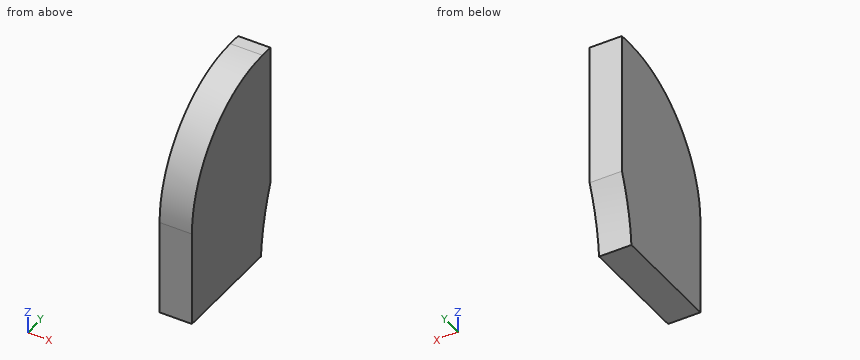
from build123d import *

# Parameters (mm, degrees)
SKETCH1_W               = 5
SKETCH1_H               = 20
BOSS_EXTRUDE1_DEPTH     = 84.5
CUT_EXTRUDE2_DEPTH      = 35
CUT_EXTRUDE2_DEPTH_BACK = 35
SKETCH5_R               = 35.5
SKETCH2_W               = 5
SKETCH2_H               = 20
CUT_EXTRUDE3_DEPTH      = 13
SKETCH8_W               = 39.75
SKETCH8_H               = 20
CUT_EXTRUDE4_DEPTH      = 13
SKETCH9_W               = 5
SKETCH9_H               = 7
CUT_EXTRUDE5_DEPTH      = 24
FILLET1_R               = 18


with BuildPart() as part:
    # Sketch1 → Boss-Extrude1 (new body)
    with BuildSketch(Plane.XY):
        with Locations((-2.5, 10)):
            Rectangle(SKETCH1_W, SKETCH1_H)
    extrude(amount=BOSS_EXTRUDE1_DEPTH)

    # Sketch5 → Cut-Extrude2 (cut, two sides: drawn at the far end of the back side and taken through both)
    with BuildSketch(Plane(origin=(0, 0, 0), x_dir=(0, 0, -1), z_dir=(1, 0, 0)).offset(-CUT_EXTRUDE2_DEPTH_BACK)):
        with Locations((-42.25, 53)):
            Circle(SKETCH5_R)
    extrude(amount=CUT_EXTRUDE2_DEPTH + CUT_EXTRUDE2_DEPTH_BACK, mode=Mode.SUBTRACT)

    # Sketch2 → Cut-Extrude3 (cut)
    with BuildSketch(Plane.ZY.offset(5)):
        with Locations((42.25, 10)):
            Rectangle(SKETCH2_W, SKETCH2_H)
    extrude(amount=-CUT_EXTRUDE3_DEPTH, mode=Mode.SUBTRACT)


with BuildPart() as cut_extrude3_piece_1:
    # of the separate pieces the step leaves, piece 1, a body of its own (cut_extrude3_pieces)
    add(part.part.solids().sort_by_distance((0, 0, 44.75))[0])

    # Sketch9 → Cut-Extrude5 (cut)
    with BuildSketch(Plane(origin=(0, 20, 0), x_dir=(1, 0, 0), z_dir=(0, 1, 0))):
        with Locations((-2.5, -81)):
            Rectangle(SKETCH9_W, SKETCH9_H)
    extrude(amount=-CUT_EXTRUDE5_DEPTH, mode=Mode.SUBTRACT)

    # Fillet1
    fillet1_edges = [cut_extrude3_piece_1.edges().sort_by_distance(p)[0] for p in [
        (-2.5, 0, 77.5),
    ]]
    fillet(fillet1_edges, radius=FILLET1_R)


with BuildPart() as cut_extrude3_piece_2:
    # of the separate pieces the step leaves, piece 2, a body of its own (cut_extrude3_pieces)
    add(part.part.solids().sort_by_distance((-5, 20, 0))[0])

    # Sketch8 → Cut-Extrude4 (cut)
    with BuildSketch(Plane.ZY.offset(5)):
        with Locations((19.875, 10)):
            Rectangle(SKETCH8_W, SKETCH8_H)
    extrude(amount=-CUT_EXTRUDE4_DEPTH, mode=Mode.SUBTRACT)


solid = cut_extrude3_piece_1.part
For this review, take the finished solid that the model builds, in its own axes (mm). Give positions to 0.01 mm unless a question says otherwise; leave off trailing zeros. Loops run counter-clockwise (first coordinate to the right, second up) from the corner with the lowest first, then second, coordinate; pieces in that order, holes last. Notation, with made-up numbers: M 31,12 L 72,12 A19 ccw 72,27 Z; hole C -11,-40 d2. An arc over 180 degrees is marked long. Put each result on its own line as item: value. Start each with the question number.
(1) For pin 1 (2 mm diameter, centred on x = -4, y = 4.5, fed in from +Z); pin 2 (1.5 mm diameter, centred on x = -2.5, y = 3.5, fed in from +Z); pin 3 (1 mm diameter, centred on x = -1.5, y = 3.5, fed in from +Z), all flat-tipped, find the tip position at first contact; note any pin that passes through.
(2) Add section C-C, the plane y = 7.5. Write out the cut boundary in (x, z).
(3) Add section B-B, the plane z = 49. Write out the cut boundary in (x, y).
(4) Add section A-A, the plane x = -1.6. Write out the cut boundary in (y, z).
(5) Wall thickness on L1, parallel to Y at x = -2.2, z = 60; L2, parallel to Z at x = -1.7, y = 5.75; L3, parallel to Y at x = -0.35, z = 67: over which ranges is each line inside the solid? List them lowest first.
Result:
1. pin 1: stops at z = 72.45
1. pin 2: stops at z = 71.12
1. pin 3: stops at z = 70.81
2. outline: M -5,44.75 L 0,44.75 L 0,74.12 L -5,74.12 Z
3. outline: M -5,0 L 0,0 L 0,18.15 L -5,18.15 Z
4. outline: M 0,44.75 L 17.59,44.75 A35.5 cw 20,55.34 L 20,77.5 L 18,77.5 A18 ccw 0,59.5 Z
5. L1: y = 0.01 to 20
5. L2: z = 44.75 to 72.69
5. L3: y = 1.64 to 20
